Autodesk Fusion 360 part; units mm, degrees
sketch "Sketch1" plane through (0, 0, 0) normal (1, 0, 0) x (0, 0, -1)
sketch "Sketch2" plane through (0, 0, 0) normal (0, 1, 0) x (1, 0, 0)
  line L0 (0, 0) -> (2.75, 0)
  line L1 (0, 0) -> (-2.75, 0)
  line L2 (0, 0) -> (5.2, 0)
  line L3 (0, 0) -> (-5.2, 0)
  circle A0 centre (-3.975, 0) radius 1.225
  circle A1 centre (3.975, 0) radius 1.225
  line L4 (5.2, 6.5) -> (-5.2, 6.5)
  line L5 (-5.2, 6.5) -> (-5.2, -6.5)
  line L6 (-5.2, -6.5) -> (5.2, -6.5)
  line L7 (5.2, -6.5) -> (5.2, 6.5)
  line L8 (5.2, 6.5) -> (-5.2, -6.5) construction
  line L9 (-5.2, 6.5) -> (5.2, -6.5) construction
  circle A2 centre (-3.975, 0) radius 0.9
  circle A3 centre (3.975, 0) radius 0.9
  dimension "d1" = 2.75
  dimension "d2" = 2.75
  dimension "d3" = 5.2
  dimension "d4" = 13
  dimension "d7" = 1.8
  dimension "d8" = 1.8
  dimension "d10" = 2.45
extrude "Extrude1" add sketch "Sketch2" along normal blind 10 contours L0 L1 L2 L3 A0 A1 L4 L5 L7 | L0 L1 L2 L3 A0 A1 L5 L6 L7 | L2 A1 A3 | L2 A1 A3 | L3 A0 A2 | L3 A0 A2
fillet "Fillet1" radius 1.202 4 edges at (-5.2, 5, 6.5) (-5.2, 5, -6.5) (5.2, 5, 6.5) (5.2, 5, -6.5)
equation "d1 = ( 5.5 / 2 ) * 1 mm"
equation "d2 = ( 5.5 / 2 ) * 1 mm"
equation "d3 = ( 10.4 / 2 ) * 1 mm"
Model file for the job. Use its own axes, mm. Give positions to 0.01 mm unless a question says otherwise; leave off trailing zeros. Order: outer loops, then holes, each group sorted by start corner. A loop starts at its lowest first (then second) coordinate and runs counter-clockwise, first axis right, second up. Notation, with made-up numbers: (40.25, 51.5) - (86.25, 51.5) arc R16 cw to (86.25, 73.5) - close; hole circle Ø11 at (50.5, -4.75). An arc over 180 degrees is marked (long way). Write item = value, one per line. Start each with the question number.
1. Probe line 1 along X through (y, z) = (5, 0) (3 decimals); line 2 along X through (y, z) = (9.5, 0.5); line 3 along Z through (x, y) = (3.5, 9). List the from-to ranges inside material, lowest first.
2. Drop a flat-ended pin along its axis: P1, Ø1.5, axis at x = -2.5, z = 0.5, coming from the -Y side. Give the stop position or say it passes through.
3. Cut at C-C, the plane x = 3.25. List the corners of the cut face in (y, z), and give its area (3 significant figures).
4. Two-plate mould, pull along X, no slides. Class faces 1 (the flat face through (5.2, 5, 0)), 2 (the flat face through (-5.2, 5, 0)), 3 (the cylindrical face through (-3.117, 4.93, 0.27)), 4 (the flat face through (0, 5, -6.5)): pulls with the +X half, pulls with the -X half, needs draft (parallel to the pull), parting line crosses it, or undercut.
5. Cut at A-A, the plane z = 0. List the corners of the cut face in (x, y) (3 decimals).
6. Cut at B-B, the plane y = 7. List the corners of the cut face in (x, z) (3 decimals).
Taken from the geometry:
q1.line_1 = -5.2 to -4.875, -3.075 to 3.075, 4.875 to 5.2
q1.line_2 = -5.2 to -4.72, -3.23 to 3.23, 4.72 to 5.2
q1.line_3 = -6.5 to -0.76, 0.76 to 6.5
q2.P1 = 0
q3.outline = (0, -6.5) - (10, -6.5) - (10, -0.53) - (0, -0.53) - close; (0, 0.53) - (10, 0.53) - (10, 6.5) - (0, 6.5) - close
q3.area = 119 mm²
q4.face_1 = pulls with the +X half
q4.face_2 = pulls with the -X half
q4.face_3 = undercut
q4.face_4 = needs draft
q5.outline = (-5.2, 0) - (-4.875, 0) - (-4.875, 10) - (-5.2, 10) - close; (-3.075, 0) - (3.075, 0) - (3.075, 10) - (-3.075, 10) - close; (4.875, 0) - (5.2, 0) - (5.2, 10) - (4.875, 10) - close
q6.outline = (-5.2, -5.298) arc R1.202 ccw to (-3.998, -6.5) - (3.998, -6.5) arc R1.202 ccw to (5.2, -5.298) - (5.2, 5.298) arc R1.202 ccw to (3.998, 6.5) - (-3.998, 6.5) arc R1.202 ccw to (-5.2, 5.298) - close; hole circle Ø1.8 at (-3.975, 0); hole circle Ø1.8 at (3.975, 0)
